Autodesk Inventor part; units mm, degrees
ref_plane "YZ Plane" through (0, 0, 0) normal (1, 0, 0) x (0, 1, 0)
ref_plane "XZ Plane" through (0, 0, 0) normal (0, 1, 0) x (-1, 0, 0)
sketch "Sketch1" plane through (0, 0, 0) normal (0, 1, 0) x (-1, 0, 0)
  circle A0 centre (0, 0) radius 62.5
  dimension "d0" = 125
extrude "Extrusion1" add sketch "Sketch1" along normal blind 20
sketch "Sketch2" plane through (0, 20, 0) normal (0, 1, 0) x (1, 0, 0)
  circle A0 centre (0, 0) radius 60
  dimension "d3" = 120
extrude "Extrusion2" cut sketch "Sketch2" against normal blind 2.5
sketch "Sketch3" plane through (0, 17.5, 0) normal (0, 1, 0) x (1, 0, 0)
  circle A0 centre (0, 0) radius 57.5
  dimension "d6" = 115
extrude "Extrusion3" cut sketch "Sketch3" against normal blind 15
sketch "Sketch4" plane through (0, 2.5, 0) normal (0, 1, 0) x (1, 0, 0)
  circle A0 centre (0, 0) radius 5
  circle A1 centre (0, 20) radius 5
  circle A2 centre (0, 40) radius 5
  circle A3 centre (20, 0) radius 5
  circle A4 centre (40, 0) radius 5
  circle A5 centre (0, -40) radius 5
  circle A6 centre (0, -20) radius 5
  circle A7 centre (-20, 0) radius 5
  circle A8 centre (-40, 0) radius 5
  dimension "d9" = 10
  dimension "d10" = 10
  dimension "d11" = 10
  dimension "d12" = 10
  dimension "d13" = 10
  dimension "d14" = 10
  dimension "d15" = 10
  dimension "d16" = 10
  dimension "d17" = 10
  dimension "d18" = 20
  dimension "d19" = 20
  dimension "d20" = 20
  dimension "d21" = 20
  dimension "d22" = 20
  dimension "d23" = 20
  dimension "d24" = 20
  dimension "d25" = 20
extrude "Extrusion4" cut sketch "Sketch4" against normal up to next
ref_plane "Work Plane1" through (0, 0, -62.5) normal (0, 0, 1) x (1, 0, 0)
sketch "Sketch5" plane through (0, 0, -62.5) normal (0, 0, 1) x (1, 0, 0)
  line L0 (62.5, 20) -> (-62.5, 20) construction
  line L1 (-62.5, 0) -> (62.5, 0) construction
  line L2 (4.25, 10) -> (-4.25, 10)
  line L3 (-4.25, 10) -> (-4.25, 5.5)
  line L4 (-4.25, 5.5) -> (4.25, 5.5)
  line L5 (4.25, 5.5) -> (4.25, 10)
  line L6 (-57.5, 2.5) -> (57.5, 2.5) construction
  line L7 (0, 0) -> (0, 20) construction
  point P0 (0, 5.5)
  dimension "d28" = 8.5
  dimension "d29" = 4.5
  dimension "d61" = 3
extrude "Extrusion5" cut sketch "Sketch5" along normal blind 17.5
sketch "Sketch6" plane through (0, 2.5, 0) normal (0, 1, 0) x (1, 0, 0)
  line L0 (0, 0) -> (50, 0) construction
  circle A0 centre (0, 0) radius 5 construction
  line L1 (0, 0) -> (35.3553, -35.3553) construction
  line L2 (0, 0) -> (50, 0) construction
  line L3 (0, 0) -> (0, -50) construction
  line L4 (0, 0) -> (35.3553, 35.3553) construction
  line L5 (0, 0) -> (50, 0) construction
  line L6 (0, 0) -> (0, 50) construction
  line L7 (0, 0) -> (-35.3553, 35.3553) construction
  line L8 (0, 0) -> (50, 0) construction
  line L9 (0, 0) -> (-50, 0) construction
  line L10 (0, 0) -> (50, 0) construction
  line L11 (0, 0) -> (-35.3553, -35.3553) construction
  line L12 (0, 0) -> (50, 0) construction
  circle A1 centre (-35.3553, 35.3553) radius 2
  circle A2 centre (0, 50) radius 2
  circle A3 centre (35.3553, 35.3553) radius 2
  circle A4 centre (50, 0) radius 2
  circle A5 centre (35.3553, -35.3553) radius 2
  circle A6 centre (0, -50) radius 2
  circle A7 centre (-35.3553, -35.3553) radius 2
  circle A8 centre (-50, 0) radius 2
  dimension "d32" = 50
  dimension "d33" = 50
  dimension "d34" = 45
  dimension "d35" = 50
  dimension "d36" = 50
  dimension "d37" = 45
  dimension "d38" = 50
  dimension "d39" = 50
  dimension "d40" = 135
  dimension "d41" = 50
  dimension "d42" = 180
  dimension "d43" = 50
  dimension "d44" = 135
  dimension "d45" = 4
  dimension "d46" = 4
  dimension "d47" = 4
  dimension "d48" = 4
  dimension "d49" = 4
  dimension "d50" = 4
  dimension "d51" = 4
  dimension "d52" = 4
extrude "Extrusion6" add sketch "Sketch6" along normal blind 17.5 contours A1 | A3 | A4 | A5 | A6 | A7 | A8
sketch "Sketch7" plane through (0, 20, 0) normal (0, 1, 0) x (1, 0, 0)
  circle A0 centre (-35.3553, -35.3553) radius 2
  circle A1 centre (35.3553, -35.3553) radius 2
  circle A2 centre (35.3553, 35.3553) radius 2
  circle A3 centre (-35.3553, 35.3553) radius 2
  circle A4 centre (50, 0) radius 2
  circle A5 centre (0, -50) radius 2
  circle A6 centre (-50, 0) radius 2
  circle A7 centre (0, 0) radius 57.5
  circle A8 centre (0, 40) radius 5
  circle A9 centre (-20, 0) radius 5
  circle A10 centre (0, -40) radius 5
  circle A11 centre (20, 0) radius 5
  circle A12 centre (0, 20) radius 5
  circle A13 centre (0, 0) radius 5
  circle A14 centre (40, 0) radius 5
  circle A15 centre (0, -20) radius 5
  circle A16 centre (-40, 0) radius 5
  circle A17 centre (0, 0) radius 62.5
  line L0 (8.9566, 60) -> (-9.0434, 60)
  line L1 (-9.0434, 60) -> (-9.0434, 17)
  line L2 (-9.0434, 17) -> (8.9566, 17)
  line L3 (8.9566, 17) -> (8.9566, 60)
  line L4 (0, 0) -> (-0.0452, 62.5) construction
  arc A18 (4.25, 62.3553) -> (-4.25, 62.3553) centre (0, 0) ccw construction
  point P0 (-0.0434, 60)
  dimension "d56" = 18
  dimension "d57" = 43
  dimension "d58" = 2.5
extrude "Extrusion7" cut sketch "Sketch7" against normal up to surface (17.5 mm away) contours L3 L2 A12 L1 A7 | A7 L1 L0 L3 | L2 A12 picked at (-7.6956, 37.9281) picked at (-1.3474, 18.3627)
equation "\"d7\" = d1 - 2 * d4"
equation "\"d10\" = d9"
equation "\"d11\" = d9"
equation "\"d12\" = d9"
equation "\"d13\" = d9"
equation "\"d14\" = d9"
equation "\"d15\" = d9"
equation "\"d16\" = d9"
equation "\"d17\" = d9"
equation "\"d19\" = d18"
equation "\"d21\" = d18"
equation "\"d23\" = d18"
equation "\"d25\" = d18"
equation "\"d33\" = d32"
equation "\"d36\" = d32"
equation "\"d38\" = d32"
equation "\"d39\" = d32"
equation "\"d41\" = d32"
equation "\"d43\" = d32"
equation "\"d46\" = d47"
equation "\"d47\" = d45"
equation "\"d48\" = d45"
equation "\"d49\" = d45"
equation "\"d50\" = d45"
equation "\"d51\" = d45"
equation "\"d52\" = d45"
equation "\"d53\" = d1 - d4"
properties part number "base bund" material "ABS Plastic"
The listing builds one solid part. Answer for the finished solid, in the listing's coordinates (mm). A direction names the side the tool comes from. Coordinates: 2 decimals unless noted, no trailing zeros. Write each loop counter-clockwise with the first axis right and the second up, starting at its lowest first coordinate (ties: lowest second). Pieces come first, ordered by that corner, then holes. Notation, with made-up numbers: (69.5, 49.25) - (124.5, 49.25) arc R23 ccw to (124.5, 77.25) - close; hole circle Ø2 at (84.25, 59). An arc over 180 degrees is marked (long way). Return JSON: item names as keys, results as strings. Group by question number.
Q1. The part is cut by section B-B on x = -20. Write down the section's boundary in (y, z), and give its area (3 significant figures).
Q2. For a pull along X with two mould halves and no side action, classify faces 3 (the flat face through (23, 20, 56)), 4 (the cylindrical face through (-33.45, 11.13, -34.75)) as +X half, -X half, draft (parallel to the pull), parting line (faces both ways), or undercut.
Q3. Find the intervals of material crossed by line 1 along Z through (x, y) = (0, 1.95); line 2 along Z through (x, y) = (0, 18.05); line 3 along Z through (x, y) = (0, 12.5), in increasing order. Write a range as [from, to].
Q4. The part is cut by section C-C on z = 20. Write down the section's boundary in (x, y).
Q5. Which of the six approach directions +Z, -Z, +X, -X, +Y, -Y give full straight-line access (tool end or side, diameter ignored) to faces 1 (the flat face through (0, 11, -60)), 2 (the flat face through (50, 20, 0))?
Q6. Flat-ended cylindrical pins translate along their axes: pin 1 Ø1 at (x, y) = (-11.5, 2.5) entering from +Z; pin 2 Ø10 at (x, z) = (45.5, 2) entering from +Y; pin 3 Ø5 at (y, z) = (14.5, 35) entering from -X; pin 4 Ø3 at (y, z) = (16, -44) entering from -X. Find the tip coordinate at first contact, or state that the pin passes through.
Q7. The part is cut by section A-A on y = 12.5. State how many separate pieces and enclosed holes the cut face has, and give its area (3 significant figures).
Evaluation:
{
 "1": {"outline": "(0, -59.21) - (20, -59.21) - (20, -56.57) - (17.5, -56.57) - (17.5, -53.91) - (2.5, -53.91) - (2.5, -5) - (0, -5) - close; (0, 5) - (2.5, 5) - (2.5, 53.91) - (17.5, 53.91) - (17.5, 56.57) - (20, 56.57) - (20, 59.21) - (0, 59.21) - close", "area": "443 mm2"},
 "2": {"face 3": "draft", "face 4": "undercut"},
 "3": {"line 1": "z = [-62.5, -45], [-35, -25], [-15, -5], [5, 15], [25, 35], [45, 62.5]", "line 2": "z = [-62.5, -60], [48, 52], [60, 62.5]", "line 3": "z = [-62.5, -60], [48, 52], [57.5, 62.5]"},
 "4": {"outline": "(-59.21, 0) - (-5, 0) - (-5, 2.5) - (-53.91, 2.5) - (-53.91, 17.5) - (-56.57, 17.5) - (-56.57, 20) - (-59.21, 20) - close; (5, 0) - (59.21, 0) - (59.21, 20) - (56.57, 20) - (56.57, 17.5) - (53.91, 17.5) - (53.91, 2.5) - (5, 2.5) - close"},
 "5": {"face 1": "+Y", "face 2": "+Z, -Z, +X, -X, +Y"},
 "6": {"pin 1": "stops at z = 61.52", "pin 2": "stops at y = 20", "pin 3": "stops at x = -53.39", "pin 4": "stops at x = -45.83"},
 "7": {"separate pieces": "8", "enclosed holes": "1", "area": "1,920 mm2"}
}
